The model under review builds one solid part; all positions refer to its coordinate system, in mm. Round coordinates to 2 decimals unless told otherwise and drop trailing zeros. Write each loop counter-clockwise with the first axis right and the second up, starting at its lowest first coordinate (ties: lowest second). Pieces come first, ordered by that corner, then holes. Notation, with made-up numbers: M 1.5,44 L 56.5,44 A13 cw 56.5,55 Z; hole C 75.5,2.25 d4. An arc over 180 degrees is marked long. One line per item, written item: value. Start each with the question number.
1) Wall thickness on probe 1 along X at (y, z) = (90, 1.3); probe 2 along X at (y, z) = (-7.5, 0.3); probe 3 along X at (y, z) = (59.5, 1.85): over which ranges is each line inside the solid? List them lowest first.
2) Take a section at A-A, the plane x = 0. State how many separate pieces and enclosed holes the cut face has, and give its area (3 significant figures).
3) Take a section at D-D, the plane y = 42.5. Write out the cut boundary in (x, z), and give its area (3 significant figures).
4) Take a section at C-C, the plane z = 1. Write out the cut boundary in (x, y), and give its area (3 significant figures).
5) Take a section at B-B, the plane y = 0. Write out the cut boundary in (x, z).
6) For P1, Ø1.5, axis at y = 48.5, z = 2, coming from the +X side; P2, Ø0.9, axis at y = 77, z = 1.5, coming from the -X side; P3, Ø1.5, axis at y = -11, z = 2, coming from the -X side, all flat-tipped, find the tip position at first contact; note any pin that passes through.
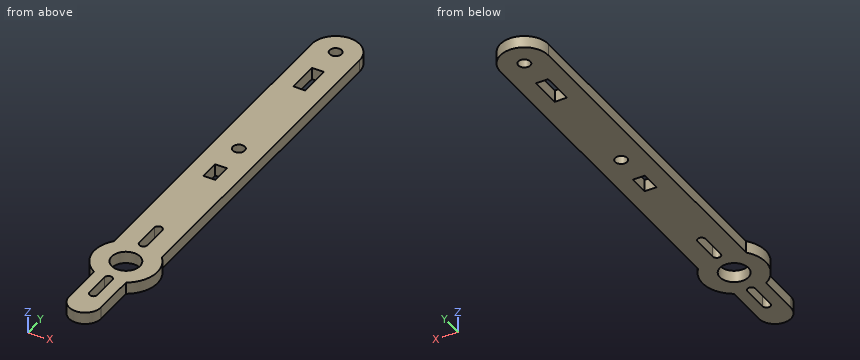
from build123d import *

# Parameters (mm, degrees)
SKETCH1_R           = 3.55
SKETCH1_R_2         = 1.5
SKETCH1_W           = 3
SKETCH1_H           = 5
SKETCH1_H_2         = 8
BOSS_EXTRUDE1_DEPTH = 3


with BuildPart() as part:
    # Sketch1 → Boss-Extrude1 (new body)
    with BuildSketch(Plane.XY):
        with BuildLine():
            Line((-6, 90), (-6, 5.139066063))
            ThreePointArc((-6, 5.139066063), (-7.791656712, -1.303873341), (-4, -6.812488532))
            Line((-4, -6.812488532), (-4, -17.5))
            ThreePointArc((-4, -17.5), (0, -21.5), (4, -17.5))
            Line((4, -17.5), (4, -6.812488532))
            ThreePointArc((4, -6.812488532), (7.791656712, -1.303873341), (6, 5.139066063))
            Line((6, 5.139066063), (6, 90))
            ThreePointArc((6, 90), (0, 96), (-6, 90))
        make_face()
        Circle(SKETCH1_R, mode=Mode.SUBTRACT)
        with Locations((0, 90)):
            Circle(SKETCH1_R_2, mode=Mode.SUBTRACT)
        with Locations((0, 48.476985236)):
            Circle(SKETCH1_R_2, mode=Mode.SUBTRACT)
        with BuildLine():
            Line((1, -7.5), (1, -13.9))
            ThreePointArc((1, -13.9), (0, -14.9), (-1, -13.9))
            Line((-1, -13.9), (-1, -7.5))
            ThreePointArc((-1, -7.5), (0, -6.5), (1, -7.5))
        make_face(mode=Mode.SUBTRACT)
        with BuildLine():
            Line((1, 7.5), (1, 13.9))
            ThreePointArc((1, 13.9), (0, 14.9), (-1, 13.9))
            Line((-1, 13.9), (-1, 7.5))
            ThreePointArc((-1, 7.5), (0, 6.5), (1, 7.5))
        make_face(mode=Mode.SUBTRACT)
        with Locations((0, 38.376985236)):
            Rectangle(SKETCH1_W, SKETCH1_H, mode=Mode.SUBTRACT)
        with Locations((0, 78.376985236)):
            Rectangle(SKETCH1_W, SKETCH1_H_2, mode=Mode.SUBTRACT)
    extrude(amount=BOSS_EXTRUDE1_DEPTH)


solid = part.part
Checked values:
1. probe 1: x = -6 to -1.5, 1.5 to 6
1. probe 2: x = -4 to -1, 1 to 4
1. probe 3: x = -6 to 6
2. separate pieces: 8
2. enclosed holes: 0
2. area: 224 mm2
3. outline: M -6,0 L 6,0 L 6,3 L -6,3 Z
3. area: 36.0 mm2
4. outline: M -6,5.14 A7.9 ccw -4,-6.81 L -4,-17.5 A4 ccw 4,-17.5 L 4,-6.81 A7.9 ccw 6,5.14 L 6,90 A6 ccw -6,90 Z; hole C 0,0 d7.1; hole M -1.5,35.88 L 1.5,35.88 L 1.5,40.88 L -1.5,40.88 Z; hole C 0,48.48 d3; hole M -1.5,74.38 L 1.5,74.38 L 1.5,82.38 L -1.5,82.38 Z; hole C 0,90 d3; hole M -1,-13.9 A1 ccw 1,-13.9 L 1,-7.5 A1 ccw -1,-7.5 Z; hole M -1,7.5 A1 ccw 1,7.5 L 1,13.9 A1 ccw -1,13.9 Z
4. area: 1,230 mm2
5. outline: M -7.9,0 L -3.55,0 L -3.55,3 L -7.9,3 Z; M 3.55,0 L 7.9,0 L 7.9,3 L 3.55,3 Z
6. P1: stops at x = 6
6. P2: stops at x = -6
6. P3: stops at x = -4
